Could you check a few things on this model? Use its own coordinates, in mm. Face numbers are marked on the shaded views. A direction names the side the tool comes from. Round coordinates to 2 decimals unless told otherwise and drop trailing zeros. Order: outer loops, then holes, each group sorted by start corner. A loop starts at its lowest first (then second) coordinate and runs counter-clockwise, first axis right, second up. Notation, with made-up numbers: (63, -22.5) -> (109, -22.5) arc R29 cw to (109, 6.5) -> close; hole circle Ø3 at (-29.75, 70). An arc over 180 degrees is marked (long way). Put each result on its own line as item: value. Start each with the question number.
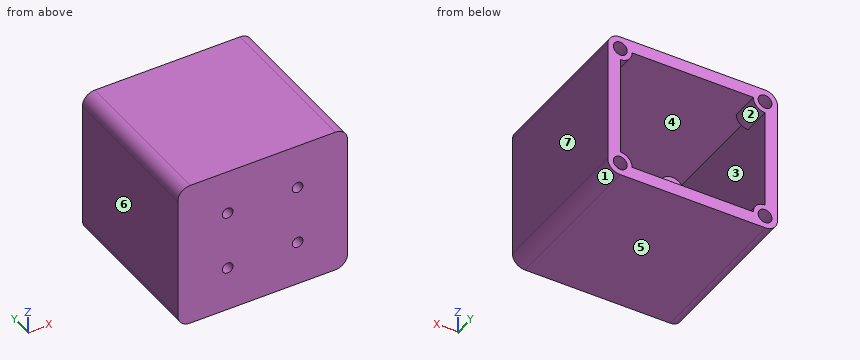
from build123d import *

# Parameters (mm, degrees)
SKETCH1_W           = 69.01
SKETCH1_H           = 60.16
BOSS_EXTRUDE3_DEPTH = 64.008
SKETCH2_W           = 58.85
SKETCH2_H           = 50
CUT_EXTRUDE4_DEPTH  = 58.928
FILLET1_R           = 5
SKETCH3_R           = 4.8067
BOSS_EXTRUDE4_DEPTH = 11.43
SKETCH3_3_R         = 2.8067
CUT_EXTRUDE5_DEPTH  = 6.35
SKETCH9_R           = 4.8067
SKETCH9_R_2         = 2.8067
BOSS_EXTRUDE5_DEPTH = 6.35
SKETCH10_R          = 2.159
CUT_EXTRUDE6_DEPTH  = 5.08
BOSS_EXTRUDE6_DEPTH = 1


with BuildPart() as part:
    # Sketch1 → Boss-Extrude3 (new body)
    with BuildSketch(Plane(origin=(0, 0, 0), x_dir=(1, 0, 0), z_dir=(0, 1, 0))):
        Rectangle(SKETCH1_W, SKETCH1_H)
    extrude(amount=BOSS_EXTRUDE3_DEPTH)

    # Sketch2 → Cut-Extrude4 (cut)
    with BuildSketch(Plane(origin=(0, 64.008, 0), x_dir=(1, 0, 0), z_dir=(0, 1, 0))):
        Rectangle(SKETCH2_W, SKETCH2_H)
    extrude(amount=-CUT_EXTRUDE4_DEPTH, mode=Mode.SUBTRACT)

    # Fillet1
    fillet1_edges = [part.edges().sort_by_distance(p)[0] for p in [
        (-34.505, 32.004, 30.08),
        (34.505, 32.004, 30.08),
        (34.505, 32.004, -30.08),
        (-34.505, 32.004, -30.08),
    ]]
    fillet(fillet1_edges, radius=FILLET1_R)

    # Sketch3 → Boss-Extrude4 (add)
    with BuildSketch(Plane(origin=(0, 64.008, 0), x_dir=(1, 0, 0), z_dir=(0, 1, 0))):
        with Locations((-29.425, 25)):
            Circle(SKETCH3_R)
        with Locations((29.425, 25)):
            Circle(SKETCH3_R)
        with Locations((-29.425, -25)):
            Circle(SKETCH3_R)
        with Locations((29.425, -25)):
            Circle(SKETCH3_R)
    extrude(amount=-BOSS_EXTRUDE4_DEPTH)

    # Sketch3<3> → Cut-Extrude5 (cut)
    with BuildSketch(Plane(origin=(0, 64.008, 0), x_dir=(1, 0, 0), z_dir=(0, 1, 0))):
        with Locations(Location((-29.425, 25, 0), (0, 0, 270))):
            Circle(SKETCH3_3_R)
        with Locations(Location((29.425, 25, 0), (0, 0, 270))):
            Circle(SKETCH3_3_R)
        with Locations(Location((29.425, -25, 0), (0, 0, 270))):
            Circle(SKETCH3_3_R)
        with Locations(Location((-29.425, -25, 0), (0, 0, 270))):
            Circle(SKETCH3_3_R)
    extrude(amount=-CUT_EXTRUDE5_DEPTH, mode=Mode.SUBTRACT)

    # Sketch9 → Boss-Extrude5 (add)
    # profile 1 of 4: a face of its own
    with BuildSketch(Plane(origin=(0, 5.08, 0), x_dir=(1, 0, 0), z_dir=(0, 1, 0))):
        with Locations(Location((-23.225, 18.85, 0), (0, 0, 90))):
            Circle(SKETCH9_R)
        with Locations(Location((-23.225, 18.85, 0), (0, 0, 270))):
            Circle(SKETCH9_R_2, mode=Mode.SUBTRACT)
    # profile 2 of 4: a face of its own
    with BuildSketch(Plane(origin=(0, 5.08, 0), x_dir=(1, 0, 0), z_dir=(0, 1, 0))):
        with Locations(Location((23.525, 19.1, 0), (0, 0, 90))):
            Circle(SKETCH9_R)
        with Locations(Location((23.525, 19.1, 0), (0, 0, 270))):
            Circle(SKETCH9_R_2, mode=Mode.SUBTRACT)
    # profile 3 of 4: a face of its own
    with BuildSketch(Plane(origin=(0, 5.08, 0), x_dir=(1, 0, 0), z_dir=(0, 1, 0))):
        with Locations(Location((23.275, -19.05, 0), (0, 0, 90))):
            Circle(SKETCH9_R)
        with Locations(Location((23.275, -19.05, 0), (0, 0, 270))):
            Circle(SKETCH9_R_2, mode=Mode.SUBTRACT)
    # profile 4 of 4: a face of its own
    with BuildSketch(Plane(origin=(0, 5.08, 0), x_dir=(1, 0, 0), z_dir=(0, 1, 0))):
        with Locations(Location((-23.475, -19.05, 0), (0, 0, 90))):
            Circle(SKETCH9_R)
        with Locations(Location((-23.475, -19.05, 0), (0, 0, 270))):
            Circle(SKETCH9_R_2, mode=Mode.SUBTRACT)
    extrude(amount=BOSS_EXTRUDE5_DEPTH)

    # Sketch10 → Cut-Extrude6 (cut)
    with BuildSketch(Plane(origin=(0, 5.08, 0), x_dir=(1, 0, 0), z_dir=(0, 1, 0))):
        with Locations(Location((14.2125, 12, 0), (0, 0, 270))):
            Circle(SKETCH10_R)
        with Locations(Location((14.2125, -12, 0), (0, 0, 270))):
            Circle(SKETCH10_R)
        with Locations(Location((-14.2125, 12, 0), (0, 0, 270))):
            Circle(SKETCH10_R)
        with Locations(Location((-14.2125, -12, 0), (0, 0, 270))):
            Circle(SKETCH10_R)
    extrude(amount=-CUT_EXTRUDE6_DEPTH, mode=Mode.SUBTRACT)

    # Sketch12 → Boss-Extrude6 (add)
    with BuildSketch(Plane(origin=(0, 5.08, 0), x_dir=(1, 0, 0), z_dir=(0, 1, 0))):
        Polygon((-26.546494391, 13.274758956), (-25.899358974, 13.274758956), (-25.899358974, 9.774758956), (-26.213461538, 9.774758956), (-26.213461538, 12.915784597), (-26.751923077, 12.915784597), align=None)
    extrude(amount=BOSS_EXTRUDE6_DEPTH)


solid = part.part
1. If we section it at B-B, the plane z = 12: Please give me the cut outline in (x, y) (1 decimal).
2. Thinking about a two-plate mould opening in X: for the marked faces 4, 5, 6 and 7, which applies, +X half, -X half, draft (parallel to the pull), parting line (faces both ways), or undercut?
3. If we section it at D-D, the plane y = 27: Please give me the cut outline in (x, z) (3 decimals), then the cut area to 3 significant figures.
4. For pin 1 Ø1.7 at (x, z) = (23, -19) entering from +Y, with a flat end and sliding along its axis, tell me the tip position at first contact or that it passes through.
5. Which directions (+Z, -Z, +X, -X, +Y, -Y) give clear straight access to the entire face, cutting with the end or side of a thin tool? Please do the marked faces 1, 2 and 3.
6. I need wall thicknesses on L1, parallel to X at y = 9, z = 19 (3 decimals); L2, parallel to X at y = 3, z = 12 (1 decimal); L3, parallel to X at y = 6.75, z = -19.1 (3 decimals). Which ranges of each line are inside material? Lowest first, please.
7. If we section it at C-C, the plane x = -8: Please give me the cut outline in (y, z), then the cut area to 3 significant figures.
8. If we section it at A-A, the plane y = 59: Please give me the cut outline in (x, z) (3 decimals).
Results below:
1. outline: (-34.5, 0) -> (-16.4, 0) -> (-16.4, 5.1) -> (-29.4, 5.1) -> (-29.4, 64) -> (-34.5, 64) -> close; (-12.1, 0) -> (12.1, 0) -> (12.1, 5.1) -> (-12.1, 5.1) -> close; (16.4, 0) -> (34.5, 0) -> (34.5, 64) -> (29.4, 64) -> (29.4, 5.1) -> (16.4, 5.1) -> close
2. face 4: undercut
2. face 5: draft
2. face 6: -X half
2. face 7: +X half
3. outline: (-34.505, -25.08) arc R5 ccw to (-29.505, -30.08) -> (29.505, -30.08) arc R5 ccw to (34.505, -25.08) -> (34.505, 25.08) arc R5 ccw to (29.505, 30.08) -> (-29.505, 30.08) arc R5 ccw to (-34.505, 25.08) -> close; hole (-29.425, -25) -> (29.425, -25) -> (29.425, 25) -> (-29.425, 25) -> close
3. area: 1,190 mm2
4. pin 1: y = 5.08
5. face 1: -Z, +X, +Y, -Y
5. face 2: +Y
5. face 3: none
6. L1: -34.505 to -29.425, -28.281 to -26.281, -20.669 to -18.669, 18.469 to 20.469, 26.081 to 28.081, 29.425 to 34.505
6. L2: -34.5 to -16.4, -12.1 to 12.1, 16.4 to 34.5
6. L3: -34.505 to -29.425, -28.025 to -26.021, -20.429 to -18.425, 18.718 to 20.718, 26.332 to 28.332, 29.425 to 34.505
7. outline: (0, -30.08) -> (64.01, -30.08) -> (64.01, -25) -> (5.08, -25) -> (5.08, 25) -> (64.01, 25) -> (64.01, 30.08) -> (0, 30.08) -> close
7. area: 904 mm2
8. outline: (-34.505, -25.08) arc R5 ccw to (-29.505, -30.08) -> (29.505, -30.08) arc R5 ccw to (34.505, -25.08) -> (34.505, 25.08) arc R5 ccw to (29.505, 30.08) -> (-29.505, 30.08) arc R5 ccw to (-34.505, 25.08) -> close; hole circle Ø5.613 at (-29.425, -25); hole circle Ø5.613 at (-29.425, 25); hole (-29.425, -20.193) arc R4.807 cw to (-24.618, -25) -> (24.618, -25) arc R4.807 cw to (29.425, -20.193) -> (29.425, 20.193) arc R4.807 cw to (24.618, 25) -> (-24.618, 25) arc R4.807 cw to (-29.425, 20.193) -> close; hole circle Ø5.613 at (29.425, -25); hole circle Ø5.613 at (29.425, 25)
